```python
from build123d import *

# Parameters (mm, degrees)
F0_R     = 11.05
F1_DEPTH = 7


with BuildPart() as f1:
    # F0 (on Top) → F1 (new body)
    with BuildSketch(Plane.XY):
        with BuildLine():
            ThreePointArc((-3.377589, 12.605332), (0, 13.05), (3.377589, 12.605332))
            Line((3.377589, 12.605332), (1.135, 17.2))
            Line((1.135, 17.2), (0, 17.2))
            Line((0, 17.2), (-1.135, 17.2))
            Line((-1.135, 17.2), (-3.377589, 12.605332))
        make_face()
        with BuildLine():
            ThreePointArc((13.000341, -1.137382), (13.037579, -0.569233), (13.05, 0))
            ThreePointArc((13.05, 0), (12.740663, 2.824537), (11.827317, 5.515168))
            ThreePointArc((11.827317, 5.515168), (11.301632, 6.525), (10.689934, 7.485172))
            ThreePointArc((10.689934, 7.485172), (8.388378, 9.99688), (5.515168, 11.827317))
            ThreePointArc((5.515168, 11.827317), (4.463363, 12.262989), (3.377589, 12.605332))
            ThreePointArc((3.377589, 12.605332), (0, 13.05), (-3.377589, 12.605332))
            ThreePointArc((-3.377589, 12.605332), (-4.463363, 12.262989), (-5.515168, 11.827317))
            ThreePointArc((-5.515168, 11.827317), (-8.388378, 9.99688), (-10.689934, 7.485172))
            ThreePointArc((-10.689934, 7.485172), (-11.301632, 6.525), (-11.827317, 5.515168))
            ThreePointArc((-11.827317, 5.515168), (-12.851741, 2.266109), (-13.000341, -1.137382))
            ThreePointArc((-13.000341, -1.137382), (-12.851741, -2.266109), (-12.605332, -3.377589))
            ThreePointArc((-12.605332, -3.377589), (-11.301632, -6.525), (-9.227743, -9.227743))
            ThreePointArc((-9.227743, -9.227743), (-8.388378, -9.99688), (-7.485172, -10.689934))
            ThreePointArc((-7.485172, -10.689934), (-4.463363, -12.262989), (-1.137382, -13.000341))
            ThreePointArc((-1.137382, -13.000341), (0, -13.05), (1.137382, -13.000341))
            ThreePointArc((1.137382, -13.000341), (4.463363, -12.262989), (7.485172, -10.689934))
            ThreePointArc((7.485172, -10.689934), (8.388378, -9.99688), (9.227743, -9.227743))
            ThreePointArc((9.227743, -9.227743), (11.301632, -6.525), (12.605332, -3.377589))
            ThreePointArc((12.605332, -3.377589), (12.851741, -2.266109), (13.000341, -1.137382))
        make_face()
        Circle(F0_R, mode=Mode.SUBTRACT)
        with BuildLine():
            ThreePointArc((5.515168, 11.827317), (8.388378, 9.99688), (10.689934, 7.485172))
            Line((10.689934, 7.485172), (11.925407, 12.4464))
            Line((11.925407, 12.4464), (11.055947, 13.175964))
            Line((11.055947, 13.175964), (10.186486, 13.905528))
            Line((10.186486, 13.905528), (5.515168, 11.827317))
        make_face()
        with BuildLine():
            ThreePointArc((11.827317, 5.515168), (12.740663, 2.824537), (13.05, 0))
            ThreePointArc((13.05, 0), (13.037579, -0.569233), (13.000341, -1.137382))
            Line((13.000341, -1.137382), (17.135784, 1.868992))
            Line((17.135784, 1.868992), (16.938693, 2.986749))
            Line((16.938693, 2.986749), (16.741603, 4.104505))
            Line((16.741603, 4.104505), (11.827317, 5.515168))
        make_face()
        with BuildLine():
            Line((15.463137, -7.617061), (12.605332, -3.377589))
            ThreePointArc((12.605332, -3.377589), (11.301632, -6.525), (9.227743, -9.227743))
            Line((9.227743, -9.227743), (14.328137, -9.582939))
            Line((14.328137, -9.582939), (14.895637, -8.6))
            Line((14.895637, -8.6), (15.463137, -7.617061))
        make_face()
        with BuildLine():
            Line((6.949298, -15.77452), (7.485172, -10.689934))
            ThreePointArc((7.485172, -10.689934), (4.463363, -12.262989), (1.137382, -13.000341))
            Line((1.137382, -13.000341), (4.816195, -16.550906))
            Line((4.816195, -16.550906), (5.882746, -16.162713))
            Line((5.882746, -16.162713), (6.949298, -15.77452))
        make_face()
        with BuildLine():
            Line((-4.816195, -16.550906), (-1.137382, -13.000341))
            ThreePointArc((-1.137382, -13.000341), (-4.463363, -12.262989), (-7.485172, -10.689934))
            Line((-7.485172, -10.689934), (-6.949298, -15.77452))
            Line((-6.949298, -15.77452), (-5.882746, -16.162713))
            Line((-5.882746, -16.162713), (-4.816195, -16.550906))
        make_face()
        with BuildLine():
            Line((-14.328137, -9.582939), (-9.227743, -9.227743))
            ThreePointArc((-9.227743, -9.227743), (-11.301632, -6.525), (-12.605332, -3.377589))
            Line((-12.605332, -3.377589), (-15.463137, -7.617061))
            Line((-15.463137, -7.617061), (-14.895637, -8.6))
            Line((-14.895637, -8.6), (-14.328137, -9.582939))
        make_face()
        with BuildLine():
            ThreePointArc((-13.000341, -1.137382), (-12.851741, 2.266109), (-11.827317, 5.515168))
            Line((-11.827317, 5.515168), (-16.741603, 4.104505))
            Line((-16.741603, 4.104505), (-16.938693, 2.986749))
            Line((-16.938693, 2.986749), (-17.135784, 1.868992))
            Line((-17.135784, 1.868992), (-13.000341, -1.137382))
        make_face()
        with BuildLine():
            ThreePointArc((-10.689934, 7.485172), (-8.388378, 9.99688), (-5.515168, 11.827317))
            Line((-5.515168, 11.827317), (-10.186486, 13.905528))
            Line((-10.186486, 13.905528), (-11.055947, 13.175964))
            Line((-11.055947, 13.175964), (-11.925407, 12.4464))
            Line((-11.925407, 12.4464), (-10.689934, 7.485172))
        make_face()
    extrude(amount=F1_DEPTH)


solid = f1.part
```
Build history of the part. All positions in model axes, mm. A direction names the side the tool comes from. Give positions to 0.01 mm unless a question says otherwise; leave off trailing zeros. Order: outer loops, then holes, each group sorted by start corner. A loop starts at its lowest first (then second) coordinate and runs counter-clockwise, first axis right, second up. Notation, with made-up numbers: M 81.25,71.25 L 125.25,71.25 A23 cw 125.25,102.25 Z; hole C 40.25,13 d2. An arc over 180 degrees is marked long. Write item = value, one per line. Start each with the question number.
(1) Slice it at D-D on y = 14.5. Write the cut outline in (x, z).
(2) Probe L1, parallel to Y at x = -1, z = 3; L2, parallel to Y at x = 2, z = 6.75; L3, parallel to X at y = 3, z = 1.25. List the from-to ranges inside material, lowest first. Write a range as [from, to].
(3) Pin check, flat tips, straight feed: pin 1 Ø2 at (x, z) = (12.5, 3.5) entering from +Y; pin 2 Ø4 at (y, z) = (-7.5, 3) entering from +X; pin 3 Ø2 at (x, z) = (-6, 1.5) entering from +Y. Stop position of each tip, or through.
(4) Slice it at C-C on y = -12. Write the cut outline in (x, z).
(5) Two-plate mould, pull along X, no slides. Class faces 6 (the flat face through (-2.241, 14.935, 3.451)), 7 (the cylindrical face through (-4.448, 12.268, 3.451)), 8 (the flat face through (-7.22, -13.2, 3.45)), 9 (the cylindrical face through (11.31, 6.51, 3.45)): released by +X, released by -X, zero draft, split by the parting line, or undercut.
(6) Which spindle directions (+Z, -Z, +X, -X, +Y, -Y) get a long thin tool onto all of the face, cutting with end or side? Do faces 1 (the flat face through (7.88, 12.88, 3.45)), 2 (the cylindrical face through (8.376, -10.007, 3.451)), 3 (the flat face through (-3, -11, 7)), 4 (the cylindrical face through (-12.855, -2.25, 3.451)), 5 (the flat face through (15.039, 0.345, 3.451)). Say none if no direction does.
(7) Slice it at B-B on y = 8. Write the cut outline in (x, z), plus the area to 3 significant figures.
(8) Slice it at A-A on x = 0. Write the cut outline in (y, z).
Responses:
q1.outline = M -2.45,0 L 2.45,0 L 2.45,7 L -2.45,7 Z
q2.L1 = [-13.01, -11], [11, 17.2]
q2.L2 = [-13.83, -10.87], [10.87, 15.43]
q2.L3 = [-16.94, -10.63], [10.63, 16.94]
q3.pin_1 = 12.8
q3.pin_2 = 15.46
q3.pin_3 = 12.49
q4.outline = M -7.35,0 L 7.35,0 L 7.35,7 L -7.35,7 Z
q5.face_6 = undercut
q5.face_7 = undercut
q5.face_8 = released by -X
q5.face_9 = released by +X
q6.face_1 = +Z, -Z, +Y
q6.face_2 = +Z, -Z, -Y
q6.face_3 = +Z, +X, -X, +Y, -Y
q6.face_4 = +Z, -Z, -X
q6.face_5 = +Z, -Z, +X
q7.outline = M -10.82,0 L -7.62,0 L -7.62,7 L -10.82,7 Z; M 7.62,0 L 10.82,0 L 10.82,7 L 7.62,7 Z
q7.area = 44.7 mm2
q8.outline = M -13.05,0 L -11.05,0 L -11.05,7 L -13.05,7 Z; M 11.05,0 L 17.2,0 L 17.2,7 L 11.05,7 Z
